from build123d import *

# Parameters (mm, degrees)
BOSS_EXTRUDE1_DEPTH = 6
BOSS_EXTRUDE2_DEPTH = 7
SKETCH4_R           = 4.7625
BOSS_EXTRUDE3_DEPTH = 15
CUT_EXTRUDE1_REACH  = 30
SKETCH5_W           = 2.4
SKETCH5_H           = 6.5
SKETCH8_W           = 9.974420143
SKETCH8_H           = 13.222039712
BOSS_EXTRUDE4_DEPTH = 37
BOSS_EXTRUDE5_DEPTH = 5
SKETCH12_R          = 4.7625
BOSS_EXTRUDE6_DEPTH = 3.5
BOSS_EXTRUDE7_DEPTH = 15
SKETCH14_W          = 83.87720003
SKETCH14_H          = 67.677452278
SKETCH14_R          = 5.7625
CUT_EXTRUDE2_DEPTH  = 5.5


with BuildPart() as part:
    # Sketch2 → Boss-Extrude1 (new body)
    with BuildSketch(Plane.XY):
        with BuildLine():
            Line((15.974420143, 6.611019856), (35.974420143, 6.611019856))
            Line((35.974420143, 6.611019856), (35.974420143, -6.611019856))
            Line((35.974420143, -6.611019856), (15.974420143, -6.611019856))
            Line((15.974420143, -6.611019856), (6.190493175, -7.51952736))
            ThreePointArc((6.190493175, -7.51952736), (0, -12.65), (-6.190493175, -7.51952736))
            Line((-6.190493175, -7.51952736), (-15.974420143, -6.611019856))
            ThreePointArc((-15.974420143, -6.611019856), (-22, 0), (-15.974420143, 6.611019856))
            Line((-15.974420143, 6.611019856), (-6.190493175, 7.51952736))
            ThreePointArc((-6.190493175, 7.51952736), (0, 12.65), (6.190493175, 7.51952736))
            Line((6.190493175, 7.51952736), (15.974420143, 6.611019856))
        make_face()
        with BuildLine():
            Line((15.604582602, 2.62815403), (2.3, 3.863579557))
            Line((2.3, 3.863579557), (2.3, 6.35))
            ThreePointArc((2.3, 6.35), (0, 8.65), (-2.3, 6.35))
            Line((-2.3, 6.35), (-2.3, 3.863579557))
            Line((-2.3, 3.863579557), (-15.604582602, 2.62815403))
            ThreePointArc((-15.604582602, 2.62815403), (-18, 0), (-15.604582602, -2.62815403))
            Line((-15.604582602, -2.62815403), (-2.3, -3.863579557))
            Line((-2.3, -3.863579557), (-2.3, -6.35))
            ThreePointArc((-2.3, -6.35), (0, -8.65), (2.3, -6.35))
            Line((2.3, -6.35), (2.3, -3.863579557))
            Line((2.3, -3.863579557), (15.604582602, -2.62815403))
            ThreePointArc((15.604582602, -2.62815403), (18, 0), (15.604582602, 2.62815403))
        make_face(mode=Mode.SUBTRACT)
    extrude(amount=BOSS_EXTRUDE1_DEPTH)

    # Sketch3 → Boss-Extrude2 (add)
    with BuildSketch(Plane(origin=(0, 0, 0), x_dir=(-1, 0, 0), z_dir=(0, 0, -1))):
        with BuildLine():
            Line((-15.974420143, -6.611019856), (-6.190493175, -7.51952736))
            ThreePointArc((-6.190493175, -7.51952736), (0, -12.65), (6.190493175, -7.51952736))
            Line((6.190493175, -7.51952736), (15.974420143, -6.611019856))
            ThreePointArc((15.974420143, -6.611019856), (22, 0), (15.974420143, 6.611019856))
            Line((15.974420143, 6.611019856), (6.190493175, 7.51952736))
            ThreePointArc((6.190493175, 7.51952736), (0, 12.65), (-6.190493175, 7.51952736))
            Line((-6.190493175, 7.51952736), (-15.974420143, 6.611019856))
            Line((-15.974420143, 6.611019856), (-35.974420143, 6.611019856))
            Line((-35.974420143, 6.611019856), (-35.974420143, -6.611019856))
            Line((-35.974420143, -6.611019856), (-15.974420143, -6.611019856))
        make_face()
    extrude(amount=BOSS_EXTRUDE2_DEPTH)

    # Sketch4 → Boss-Extrude3 (add)
    with BuildSketch(Plane(origin=(0, 0, -7), x_dir=(-1, 0, 0), z_dir=(0, 0, -1))):
        with Locations(Location((0, 0, 0), (0, 0, 90))):  # turned: the seam where the file's is
            Circle(SKETCH4_R)
    extrude(amount=BOSS_EXTRUDE3_DEPTH)

    # Sketch5 → Cut-Extrude1 (cut, up to next)
    with BuildSketch(Plane(origin=(0, 0, -22), x_dir=(-1, 0, 0), z_dir=(0, 0, -1)), mode=Mode.PRIVATE) as cut_extrude1_sk1:
        Rectangle(SKETCH5_W, SKETCH5_H)
    cut_extrude1_tool1 = extrude(cut_extrude1_sk1.sketch, amount=-CUT_EXTRUDE1_REACH, mode=Mode.PRIVATE) & part.part
    add(cut_extrude1_tool1.solids().sort_by_distance((0, 0, -22))[0], mode=Mode.SUBTRACT)

    # Sketch8 → Boss-Extrude4 (add)
    with BuildSketch(Plane.XY.offset(6)):
        with Locations((30.987210072, 0)):
            Rectangle(SKETCH8_W, SKETCH8_H)
    extrude(amount=BOSS_EXTRUDE4_DEPTH)

    # Sketch10 → Boss-Extrude5 (add)
    with BuildSketch(Plane.XY.offset(43)):
        Polygon((35.974420143, 6.611019856), (15.974420143, 6.611019856), (6.190493175, 7.51952736), (-6.190493175, 7.51952736), (-6.190493175, -7.51952736), (6.190493175, -7.51952736), (15.974420143, -6.611019856), (35.974420143, -6.611019856), align=None)
    extrude(amount=BOSS_EXTRUDE5_DEPTH)

    # Sketch12 → Boss-Extrude6 (add)
    with BuildSketch(Plane.XY.offset(48)):
        with Locations(Location((0, 0, 0), (0, 0, 90))):  # turned: the seam where the file's is
            Circle(SKETCH12_R)
    extrude(amount=BOSS_EXTRUDE6_DEPTH)

    # Sketch13 → Boss-Extrude7 (add)
    with BuildSketch(Plane.XY.offset(51.5)):
        Polygon((3.75277675, 0), (1.876388375, 3.25), (-1.876388375, 3.25), (-3.75277675, 0), (-1.876388375, -3.25), (1.876388375, -3.25), align=None)
    extrude(amount=BOSS_EXTRUDE7_DEPTH)

    # Sketch14 → Cut-Extrude2 (cut)
    with BuildSketch(Plane(origin=(0, 0, -7), x_dir=(-1, 0, 0), z_dir=(0, 0, -1))):
        with Locations((-8.599932489, 1.250992594)):
            Rectangle(SKETCH14_W, SKETCH14_H)
        with BuildLine():
            Line((-35.974420143, -6.611019856), (-15.974420143, -6.611019856))
            Line((-15.974420143, -6.611019856), (-6.190493175, -7.51952736))
            ThreePointArc((-6.190493175, -7.51952736), (0, -12.65), (6.190493175, -7.51952736))
            Line((6.190493175, -7.51952736), (15.974420143, -6.611019856))
            ThreePointArc((15.974420143, -6.611019856), (22, 0), (15.974420143, 6.611019856))
            Line((15.974420143, 6.611019856), (6.190493175, 7.51952736))
            ThreePointArc((6.190493175, 7.51952736), (0, 12.65), (-6.190493175, 7.51952736))
            Line((-6.190493175, 7.51952736), (-15.974420143, 6.611019856))
            Line((-15.974420143, 6.611019856), (-35.974420143, 6.611019856))
            Line((-35.974420143, 6.611019856), (-35.974420143, -6.611019856))
        make_face(mode=Mode.SUBTRACT)
        with BuildLine():
            Line((-35.974420143, 6.611019856), (-35.974420143, -6.611019856))
            Line((-35.974420143, -6.611019856), (-15.974420143, -6.611019856))
            Line((-15.974420143, -6.611019856), (-6.190493175, -7.51952736))
            ThreePointArc((-6.190493175, -7.51952736), (0, -12.65), (6.190493175, -7.51952736))
            Line((6.190493175, -7.51952736), (15.974420143, -6.611019856))
            ThreePointArc((15.974420143, -6.611019856), (22, 0), (15.974420143, 6.611019856))
            Line((15.974420143, 6.611019856), (6.190493175, 7.51952736))
            ThreePointArc((6.190493175, 7.51952736), (0, 12.65), (-6.190493175, 7.51952736))
            Line((-6.190493175, 7.51952736), (-15.974420143, 6.611019856))
            Line((-15.974420143, 6.611019856), (-35.974420143, 6.611019856))
        make_face()
        with Locations(Location((0, 0, 0), (0, 0, 90))):  # turned: the seam where the file's is
            Circle(SKETCH14_R, mode=Mode.SUBTRACT)
    extrude(amount=-CUT_EXTRUDE2_DEPTH, mode=Mode.SUBTRACT)


solid = part.part
Input: part model. Units: mm. Frame: model coordinates. A direction names the side the tool comes from. Give positions to 0.01 mm unless a question says otherwise; leave off trailing zeros. Order: outer loops, then holes, each group sorted by start corner. A loop starts at its lowest first (then second) coordinate and runs counter-clockwise, first axis right, second up. Notation, with made-up numbers: (73.5, 82) - (113.5, 82) arc R29 cw to (113.5, 119) - close; hole circle Ø3 at (55, 77.5). An arc over 180 degrees is marked (long way). Answer as a JSON object with one key per item and string values. Group by question number.
Q1. Line query: probe 1 along Z at (x, y) = (7, -3.5); probe 2 along X at (y, z) = (0, -12); probe 3 along Z at (x, y) = (1.5, 1.25). Output: solid intervals per line, ascending.
Q2. First-contact query: pin 1 Ø10 at (x, z) = (25, 36) entering from +Y; pin 2 Ø0.7 at (y, z) = (-5, 2) entering from -X; pin 3 Ø12 at (x, y) = (11, -2) entering from -Z; pin 4 Ø1.5 at (x, z) = (16.5, 50.5) entering from -Y. Flat tips, straight axial feed; report the tip coordinate or a pass-through.
Q3. Set-up query: faces 4 (the face through (10, 0, 43)), 5 (the face through (1.2, 0, -11)), 6 (the face through (0, -3.25, 59)), 7 (the face through (3, 2, 51.5)), 8 (the face through (-0.05, -8.65, 2.96)). Return all of +Z, -Z, +X, -X, +Y, -Y with unobstructed straight access to the full face (end or side cutting, diameter ignored); none if empty.
Q4. Mould query, pull axis Y, two halves, no side actions, for faces 1 (the face through (26, 0, 24)), 2 (the face through (-2.83, -1.6, 58.9)), 3 (the face through (2.3, 5, 3)). Classes: pulls with the +Y half, pulls with the -Y half, needs draft (parallel to the pull), parting line crosses it, or undercut.
Q5. Cut plane D-D, the plane z = 17. Output: boundary loops of the cut face in (x, y), then the cut area to 3 significant figures.
Q6. Cut plane C-C, the plane x = -11.5. Output: boundary loops of the cut face in (y, z), then the cut area to 3 significant figures.
Q7. Cut plane A-A, the plane x = 0. Count the separate pieces of the cut face and the enclosed holes in it, then the cut area to 3 significant figures.
Results:
{
 "1": {"probe 1": "-1.5 to 6, 43 to 48", "probe 2": "-4.76 to -1.2, 1.2 to 4.76", "probe 3": "-22 to 0, 43 to 66.5"},
 "2": {"pin 1": "y = 6.61", "pin 2": "x = -20.1", "pin 3": "z = -7", "pin 4": "through"},
 "3": {"face 4": "-X, +Y, -Y", "face 5": "-Z", "face 6": "+Z, +X, -X, -Y", "face 7": "+Z", "face 8": "none"},
 "4": {"face 1": "needs draft", "face 2": "pulls with the -Y half", "face 3": "undercut"},
 "5": {"outline": "(26, -6.61) - (35.97, -6.61) - (35.97, 6.61) - (26, 6.61) - close", "area": "132 mm^2"},
 "6": {"outline": "(-7.03, -1.5) - (7.03, -1.5) - (7.03, 6) - (3.01, 6) - (3.01, 0) - (-3.01, 0) - (-3.01, 6) - (-7.03, 6) - close", "area": "69.3 mm^2"},
 "7": {"separate pieces": "3", "enclosed holes": "0", "area": "355 mm^2"}
}
